from build123d import *

# Parameters (mm, degrees)
F0_W     = 3.175
F0_H     = 40.64
F1_DEPTH = 63.5


with BuildPart() as f1:
    # F0 (on Front) → F1 (new body)
    with BuildSketch(Plane.XZ):
        Polygon((48.5775, -3.175), (48.5775, 3.175), (45.4025, 3.175), (25.0825, 3.175), (21.9075, 3.175), (1.5875, 3.175), (-1.5875, 3.175), (-21.9075, 3.175), (-25.0825, 3.175), (-45.4025, 3.175), (-48.5775, 3.175), (-48.5775, -3.175), align=None)
        with Locations((46.99, 23.495)):
            Rectangle(F0_W, F0_H)
        with Locations((23.495, 23.495)):
            Rectangle(F0_W, F0_H)
        with Locations((-46.99, 23.495)):
            Rectangle(F0_W, F0_H)
        with Locations((0, 23.495)):
            Rectangle(F0_W, F0_H)
        with Locations((-23.495, 23.495)):
            Rectangle(F0_W, F0_H)
    extrude(amount=F1_DEPTH)


solid = f1.part
Geometry check sheet. Reference: the model listing, model coordinates, mm. A direction names the side the tool comes from. Round coordinates to 2 decimals unless told otherwise and drop trailing zeros. Write each loop counter-clockwise with the first axis right and the second up, starting at its lowest first coordinate (ties: lowest second). Pieces come first, ordered by that corner, then holes. Notation, with made-up numbers: (38.5, 27) -> (45.5, 27) arc R36 ccw to (45.5, 65) -> close; hole circle Ø5 at (18.25, -37.5). An arc over 180 degrees is marked (long way). One line per item, written item: value. Start each with the question number.
(1) Cross-section at C-C, the plane x = -29. Record the cut outline in (y, z) (3 decimals), and give its area (3 significant figures).
(2) Draft check along X on faces 3 (the flat face through (-12, -31, 3.175)), 4 (the flat face through (48.578, -31, 20)), 5 (the flat face through (0, -31, 43.815)). Enter one of: +X half, -X half, draft (parallel to the pull), parting line (faces both ways), or undercut.
(3) Cross-section at A-A, the plane z = 12. Record the cut outline in (x, y).
(4) Scan lines: line 1 (X direction, y = -19.5, z = 35); line 2 (Z direction, x = 29.5, y = -53.5) (3 decimals). Record each from-to range of solid material in increasing order. Write a range as [from, to].
(5) Cross-section at B-B, the plane y = -48. Record the cut outline in (x, z) (1 decimal), and give its area (3 significant figures).
(6) Access from +Z, -Z, +X, -X, +Y, -Y to the whole of each face (thin tool, end or side, straight path). Record for faces 1 (the flat face through (-48.578, -31, 21)), 2 (the flat face through (21.908, -31, 23)).
(7) Go/stop test with flat-tipped pins: pin 1 Ø10 at (x, y) = (-9, -28.5) entering from +Z (3 decimals); pin 2 Ø16.5 at (x, y) = (15, -38.5) entering from +Z (3 decimals). Record where each tip stops, or that it passes through.
Answer:
1. outline: (-63.5, -3.175) -> (0, -3.175) -> (0, 3.175) -> (-63.5, 3.175) -> close
1. area: 403 mm²
2. face 3: undercut
2. face 4: +X half
2. face 5: draft
3. outline: (-48.58, -63.5) -> (-45.4, -63.5) -> (-45.4, 0) -> (-48.58, 0) -> close; (-25.08, -63.5) -> (-21.91, -63.5) -> (-21.91, 0) -> (-25.08, 0) -> close; (-1.59, -63.5) -> (1.59, -63.5) -> (1.59, 0) -> (-1.59, 0) -> close; (21.91, -63.5) -> (25.08, -63.5) -> (25.08, 0) -> (21.91, 0) -> close; (45.4, -63.5) -> (48.58, -63.5) -> (48.58, 0) -> (45.4, 0) -> close
4. line 1: [-48.58, -45.4], [-25.08, -21.91], [-1.59, 1.59], [21.91, 25.08], [45.4, 48.58]
4. line 2: [-3.175, 3.175]
5. outline: (-48.6, -3.2) -> (48.6, -3.2) -> (48.6, 43.8) -> (45.4, 43.8) -> (45.4, 3.2) -> (25.1, 3.2) -> (25.1, 43.8) -> (21.9, 43.8) -> (21.9, 3.2) -> (1.6, 3.2) -> (1.6, 43.8) -> (-1.6, 43.8) -> (-1.6, 3.2) -> (-21.9, 3.2) -> (-21.9, 43.8) -> (-25.1, 43.8) -> (-25.1, 3.2) -> (-45.4, 3.2) -> (-45.4, 43.8) -> (-48.6, 43.8) -> close
5. area: 1,260 mm²
6. face 1: +Z, -Z, -X, +Y, -Y
6. face 2: +Z, +Y, -Y
7. pin 1: z = 3.175
7. pin 2: z = 43.815
